Read the model definition and answer for the solid it produces. Units are mm, in the model's axes. A direction names the side the tool comes from. Give positions to 0.01 mm unless a question says otherwise; leave off trailing zeros. Write each loop counter-clockwise with the first axis right and the second up, starting at its lowest first coordinate (ties: lowest second). Pieces come first, ordered by that corner, then holes.
```python
from build123d import *

# Parameters (mm, degrees)
SKETCH1_R           = 75
BOSS_EXTRUDE1_DEPTH = 12
SKETCH2_R           = 5
CUT_EXTRUDE1_DEPTH  = 107.742681248
SKETCH3_R           = 10
CUT_EXTRUDE2_DEPTH  = 11.873117
CIRPATTERN1_START   = 0.12688314
CIRPATTERN1_DEPTH   = 11.87311686


# Read off the part's stored shape, not the designer's step: CirPattern1
with BuildPart() as part:
    # Sketch1 → Boss-Extrude1 (new body)
    with BuildSketch(Plane(origin=(0, 0, 0), x_dir=(1, 0, 0), z_dir=(0, 1, 0))):
        with Locations(Location((0, 0, 0), (0, 0, 270))):
            Circle(SKETCH1_R)
    extrude(amount=BOSS_EXTRUDE1_DEPTH)

    # Sketch2 → Cut-Extrude1 (cut, through all)
    with BuildSketch(Plane(origin=(0, 0, 0), x_dir=(1, 0, 0), z_dir=(0, 1, 0))):
        with Locations(Location((0, 0, 0), (0, 0, 270))):
            Circle(SKETCH2_R)
    extrude(amount=CUT_EXTRUDE1_DEPTH, mode=Mode.SUBTRACT)

    # Sketch3 → Cut-Extrude2 (cut)
    with BuildSketch(Plane(origin=(0, 12, 0), x_dir=(1, 0, 0), z_dir=(0, 1, 0))):
        with Locations((-13.924696634, 0)):
            Circle(SKETCH3_R)
    extrude(amount=-CUT_EXTRUDE2_DEPTH, mode=Mode.SUBTRACT)

    # CirPattern1 outline → CirPattern1 (cut)
    with BuildSketch(Plane(origin=(0, 0, 0), x_dir=(1, 0, 0), z_dir=(0, 1, 0)).offset(CIRPATTERN1_START)):
        with BuildLine():
            ThreePointArc((4.983656749, -0.403937386), (4.045084972, -2.938926261), (1.924201913, -4.614915709))
            ThreePointArc((1.924201913, -4.614915709), (1.809639041, -4.930477322), (1.705733075, -5.249706602))
            ThreePointArc((1.705733075, -5.249706602), (1.434033119, -5.052519084), (1.155867346, -4.864562743))
            ThreePointArc((1.155867346, -4.864562743), (-1.545084972, -4.755282581), (-3.794434565, -3.256112149))
            ThreePointArc((-3.794434565, -3.256112149), (-4.129953368, -3.244670285), (-4.465667165, -3.244497111))
            ThreePointArc((-4.465667165, -3.244497111), (-8.046844111, -8.090169944), (-13.76199737, -9.99867636))
            ThreePointArc((-13.76199737, -9.99867636), (-7.393137845, -22.753738634), (5.256615242, -16.178198193))
            ThreePointArc((5.256615242, -16.178198193), (19.355486162, -14.062583847), (17.010764256, 0))
            ThreePointArc((17.010764256, 0), (19.355486162, 14.062583847), (5.256615242, 16.178198193))
            ThreePointArc((5.256615242, 16.178198193), (-7.393137845, 22.753738634), (-13.76199737, 9.99867636))
            ThreePointArc((-13.76199737, 9.99867636), (-8.046844111, 8.090169944), (-4.465667165, 3.244497111))
            ThreePointArc((-4.465667165, 3.244497111), (-4.129953368, 3.244670285), (-3.794434565, 3.256112149))
            ThreePointArc((-3.794434565, 3.256112149), (-1.545084972, 4.755282581), (1.155867346, 4.864562743))
            ThreePointArc((1.155867346, 4.864562743), (1.434033119, 5.052519084), (1.705733075, 5.249706602))
            ThreePointArc((1.705733075, 5.249706602), (1.809639041, 4.930477322), (1.924201913, 4.614915709))
            ThreePointArc((1.924201913, 4.614915709), (4.045084972, 2.938926261), (4.983656749, 0.403937386))
            ThreePointArc((4.983656749, 0.403937386), (5.248371803, 0.197467719), (5.519868181, 0))
            ThreePointArc((5.519868181, 0), (5.248371803, -0.197467719), (4.983656749, -0.403937386))
        make_face()
    extrude(amount=CIRPATTERN1_DEPTH, mode=Mode.SUBTRACT)


solid = part.part
```
Item 1: Section B-B (x = -16.5) is taken. Write down the section's boundary in (y, z).
Result set:
outline: (0, -73.16) - (12, -73.16) - (12, -9.66) - (0.13, -9.66) - (0.13, 9.66) - (12, 9.66) - (12, 73.16) - (0, 73.16) - close
Item 2: Find the intervals of material crossed by line 1 along Z through (x, y) = (20, 6); line 2 along Z through (x, y) = (-0.5, 10.5); line 3 along X through (y, z) = (8, 2), in increasing order.
Result set:
line 1: z = -72.28 to -13.05, -3.32 to 3.32, 13.05 to 72.28
line 2: z = -75 to -22.49, 22.49 to 75
line 3: x = -74.97 to -23.72, 19.12 to 74.97
Item 3: Section A-A (y = 3.25) is taken. Write down the section's boundary in (x, z).
Result set:
outline: circle Ø150 at (0, 0); (-4.47, -3.24) arc R10 cw to (-3.79, -3.26) arc R5 cw to (-4.27, -2.6) arc R10 cw to start; (-4.47, 3.24) arc R10 cw to (-4.27, 2.6) arc R5 cw to (-3.79, 3.26) arc R10 cw to start; (1.16, -4.86) arc R10 cw to (1.71, -5.25) arc R10 cw to (1.92, -4.61) arc R5 cw to start; (1.16, 4.86) arc R5 cw to (1.92, 4.61) arc R10 cw to (1.71, 5.25) arc R10 cw to start; (4.98, -0.4) arc R10 cw to (5.52, 0) arc R10 cw to (4.98, 0.4) arc R5 cw to start; hole (-13.76, -10) arc R10 ccw (long way) to (5.26, -16.18) arc R10 ccw (long way) to (17.01, 0) arc R10 ccw (long way) to (5.26, 16.18) arc R10 ccw (long way) to (-13.76, 10) arc R10 ccw (long way) to start
Item 4: Each of these flat-tipped pins is pushed along its axis until it touches: pin 1 Ø3 at (y, z) = (9.5, -49) entering from -X; pin 2 Ø3 at (x, y) = (-37, 3) entering from +Z; pin 3 Ø1.5 at (x, y) = (-13, 10) entering from +Z; pin 4 Ø8 at (x, z) = (0, 0) entering from -Y. Where does it stop, or does it pass through?
Result set:
pin 1: stops at x = -58.04
pin 2: stops at z = 66.07
pin 3: stops at z = 73.99
pin 4: passes through
Item 5: Which of the six approach directions +Z, -Z, +X, -X, +Y, -Y give full straight-line access (tool end or side, diameter ignored) to faces 1 (the cylindrical face through (19.223, 5.98, 14.241)), 2 (the cylindrical face through (5, 6, 0))?
Result set:
face 1: +Y
face 2: +Y, -Y
Item 6: Determine the mould class of faces 3 (the cylindrical face through (19.484, 5.98, -13.881)), 4 (the flat face through (-16, 0, 16)), 5 (the cylindrical face through (-45.636, 5.916, -59.517)) for opening direction Z: pulls with the +Z half, pulls with the -Z half, needs draft (parallel to the pull), parting line crosses it, or undercut.
Result set:
face 3: undercut
face 4: needs draft
face 5: parting line crosses it
Item 7: Section C-C (z = -7.5) is taken. Write down the section's boundary in (x, y).
Result set:
outline: (-74.62, 0) - (74.62, 0) - (74.62, 12) - (21.24, 12) - (21.24, 0.13) - (-20.54, 0.13) - (-20.54, 12) - (-74.62, 12) - close
Item 8: Section D-D (z = -40.5) is taken. Write down the section's boundary in (x, y).
Result set:
outline: (-63.12, 0) - (63.12, 0) - (63.12, 12) - (-63.12, 12) - close
